```python
from build123d import *

# Parameters (mm, degrees)
F0_R     = 11
F0_W     = 50
F0_H     = 80
F0_R_2   = 7.5
F0_H_2   = 5
F0_R_3   = 4
F1_DEPTH = 10
F2_DEPTH = 60
F3_DEPTH = 10
F4_DEPTH = 25
F5_R     = 1
F6_DEPTH = 25


with BuildPart() as f1:
    # F0 (on Top) → F1 (new body)
    with BuildSketch(Plane.XY):
        with BuildLine():
            Line((-25, 22.8104994827), (-25, -92.1895005173))
            ThreePointArc((-25, -92.1895005173), (0, -117.1895005173), (25, -92.1895005173))
            Line((25, -92.1895005173), (25, 22.8104994827))
            Line((25, 22.8104994827), (-25, 22.8104994827))
        make_face()
        with Locations((0, -92.1895005173)):
            Circle(F0_R, mode=Mode.SUBTRACT)
        with Locations((0, 67.8104994827)):
            Rectangle(F0_W, F0_H)
        with Locations((0, 92.8104994827)):
            Circle(F0_R_2, mode=Mode.SUBTRACT)
        with Locations((0, 25.3104994827)):
            Rectangle(F0_W, F0_H_2)
        with Locations((0, 92.8104994827)):
            Circle(F0_R_2)
        with Locations((0, 92.8104994827)):
            Circle(F0_R_3, mode=Mode.SUBTRACT)
        with Locations((0, 92.8104994827)):
            Circle(F0_R_3)
    extrude(amount=F1_DEPTH)

    # F0 (on Top) → F2 (join)
    with BuildSketch(Plane.XY):
        with Locations((0, 25.3104994827)):
            Rectangle(F0_W, F0_H_2)
    extrude(amount=-F2_DEPTH)

    # F0 (on Top) → F3 (join)
    with BuildSketch(Plane.XY):
        with Locations((0, 92.8104994827)):
            Circle(F0_R_2)
        with Locations((0, 92.8104994827)):
            Circle(F0_R_3, mode=Mode.SUBTRACT)
    extrude(amount=-F3_DEPTH)

    # F0 (on Top) → F4 (join)
    with BuildSketch(Plane.XY):
        with Locations((0, 92.8104994827)):
            Circle(F0_R_3)
    extrude(amount=-F4_DEPTH)

    # F5 (on face) → F6 (cut)
    with BuildSketch(Plane(origin=(0, 27.8104994827, 0), x_dir=(-1, 0, 0), z_dir=(0, 1, 0))):
        with Locations((-12.5, -25)):
            Circle(F5_R)
        with Locations((12.5, -25)):
            Circle(F5_R)
        with Locations((-12.5, -50)):
            Circle(F5_R)
        with Locations((12.5, -50)):
            Circle(F5_R)
    extrude(amount=-F6_DEPTH, mode=Mode.SUBTRACT)


solid = f1.part
```
CAD build for the part. Positions are in the model's coordinates, mm. A direction names the side the tool comes from. Coordinates: 2 decimals unless noted, no trailing zeros. Order: outer loops, then holes, each group sorted by start corner. A loop starts at its lowest first (then second) coordinate and runs counter-clockwise, first axis right, second up. Notation, with made-up numbers: M 68,30 L 73,30 A33 ccw 73,66 Z; hole C 47,71 d2. An arc over 180 degrees is marked long. Write each question's results on one line, items separated by ' | '. Start each with the question number.
Q1. Cut at C-C (z = -22). List the corners of the cut face in (x, y), then the cut area to 3 significant figures.
Q2. Cut at B-B (x = 0). List the corners of the cut face in (y, z), then the cut area to 3 significant figures.
Q3. Flat gauge pins, fed straight in: P1, Ø2.5, axis at x = -12.5, z = -50, coming from the -Y side; P2, Ø9, axis at x = 0, y = 91.5, coming from the -Z side; P3, Ø15, axis at x = 0, y = 79, coming from the -Z side; P4, Ø20, axis at x = 0, y = -92.19, coming from the +Z side. Where does each tip first touch, or does it go through?
Q4. Pull direction X, two halves, no side cores. Call faces 6 (the flat face through (0, 68, 0)), 7 (the flat face through (-25, 8, 1)), 8 (the cylindrical face through (-0.55, -117.183, 4.93)), 9 (the cylindrical face through (-8.73, -98.88, 4.93)): +X half, -X half, draft (parallel to the pull), parting line (faces both ways), or undercut.
Q5. Cut at A-A (z = 2). List the corners of the cut face in (x, y), then the cut area to 3 significant figures.
Q6. Cut at D-D (x = -20.5). List the corners of the cut face in (y, z).
Q7. Drill centre lines: probe 1 along Z at (x, y) = (-12.5, 25.4); probe 2 along Z at (x, y) = (12, 26); probe 3 along Y at (x, z) = (0, 6.75). Where is each one in solid material? Low to high. Write a range as from..to.
Q8. Which spindle directions (+Z, -Z, +X, -X, +Y, -Y) get a long thin tool onto all of the face, cutting with end or side? Do faces 1 (the flat face through (0, -46, 0)), 2 (the flat face through (0, 93, -25)), 3 (the flat face through (0, 107.81, 5)), 4 (the flat face through (0, 25, -60)), 5 (the cylindrical face through (-0.521, 96.776, -17.395)). Say none if no direction does.
Found:
1) outline: M -25,22.81 L 25,22.81 L 25,27.81 L -25,27.81 Z; C 0,92.81 d8 | area: 300 mm²
2) outline: M -117.19,0 L -103.19,0 L -103.19,10 L -117.19,10 Z; M -81.19,0 L 22.81,0 L 22.81,-60 L 27.81,-60 L 27.81,0 L 85.31,0 L 85.31,-10 L 88.81,-10 L 88.81,-25 L 96.81,-25 L 96.81,-10 L 100.31,-10 L 100.31,0 L 107.81,0 L 107.81,10 L -81.19,10 Z | area: 2,600 mm²
3) P1: y = 22.81 | P2: z = -25 | P3: z = -10 | P4: through
4) face 6: draft | face 7: -X half | face 8: parting line | face 9: undercut
5) outline: M -25,-92.19 A25 ccw 25,-92.19 L 25,107.81 L -25,107.81 Z; hole C 0,-92.19 d22 | area: 10,600 mm²
6) outline: M -106.5,0 L 22.81,0 L 22.81,-60 L 27.81,-60 L 27.81,0 L 107.81,0 L 107.81,10 L -106.5,10 Z
7) probe 1: -60..-51, -49..-26, -24..10 | probe 2: -60..-50.87, -49.13..-25.87, -24.13..10 | probe 3: -117.19..-103.19, -81.19..107.81
8) face 1: -Z, +X, -X, -Y | face 2: -Z, +X, -X, +Y | face 3: +Z, -Z, +X, -X, +Y | face 4: -Z, +X, -X, +Y, -Y | face 5: -Z
